Geometry check sheet. Reference: the model listing, model coordinates, mm. A direction names the side the tool comes from. Round coordinates to 2 decimals unless told otherwise and drop trailing zeros. Order: outer loops, then holes, each group sorted by start corner. A loop starts at its lowest first (then second) coordinate and runs counter-clockwise, first axis right, second up. Notation, with made-up numbers: (23, -33.75) - (30, -33.75) arc R22 ccw to (30, 3.25) - close; hole circle Ø10 at (83, 11). An arc over 180 degrees is marked (long way). Return JSON: item names as keys, results as strings. Group by question number.
Q1. Sectioned sample at B-B, the plane y = 1. Record the cut outline in (x, z).
Q2. Sectioned sample at A-A, the plane x = 0. Record the cut outline in (y, z) (3 decimals).
Q3. Tool access check on faces 1 (the flat face through (48.26, 0, 3)), 2 (the flat face through (1, -54.483, 3)), 3 (the flat face through (-61, 3.175, 3)). Record the directions out of +Z, -Z, +X, -X, +Y, -Y that give a thin tool (end or side, any length) a straight path to the whole face; none if there is none.
Q4. Draft check along Y on faces 4 (the cylindrical face through (0.62, -54.65, 3.13)), 5 (the flat face through (-39, 6, 6.35)), 6 (the cylindrical face through (-1.575, -73.643, 3.131)), 7 (the cylindrical face through (1.575, 73.643, 3.131)). Enter one of: pulls with the +Y half, pulls with the -Y half, needs draft (parallel to the pull), parting line crosses it, or undercut.
Q5. Sectioned sample at C-C, the plane x = -55.5. Record the cut outline in (y, z) (3 decimals).
Q6. Gauge pin test, flat ends, axial feed: pin 1 Ø5.5 at (x, y) = (0, -59.37) entering from -Z; pin 2 Ø1.9 at (x, z) = (16, 1.5) entering from +Y; pin 3 Ø1.9 at (x, z) = (-6.5, 3) entering from -Y; pin 4 Ø1.9 at (x, z) = (-55, 2) entering from -Y. Record the tip position at first contact, or that the pin passes through.
Q7. Material ranges on line 1 along X through (y, z) = (-1, 1.25); line 2 along X through (y, z) = (57, 2); line 3 along Y through (x, z) = (65, 1.75) (1 decimal), recorded low to high.
```python
from build123d import *

# Parameters (mm, degrees)
SKETCH1_R           = 73.66
BOSS_EXTRUDE1_DEPTH = 6.35
CUT_EXTRUDE1_DEPTH  = 7.35
SKETCH4_R           = 4.7625
CUT_EXTRUDE2_DEPTH  = 7.35
SKETCH5_W           = 76.2
SKETCH5_H           = 108.966
CUT_EXTRUDE5_DEPTH  = 7.35


with BuildPart() as part:
    # Sketch1 → Boss-Extrude1 (new body)
    with BuildSketch(Plane.XY):
        Circle(SKETCH1_R)
    extrude(amount=BOSS_EXTRUDE1_DEPTH)

    # Sketch2 → Cut-Extrude1 (cut, through all)
    with BuildSketch(Plane(origin=(0, 0, 0), x_dir=(-1, 0, 0), z_dir=(0, 0, -1))):
        Polygon((-48.26, 0), (-48.26, 3.175), (-76.2, 3.175), (-76.2, -3.175), (-48.26, -3.175), align=None)
        Polygon((48.26, -3.175), (48.26, 0), (48.26, 3.175), (76.2, 3.175), (76.2, -3.175), align=None)
    extrude(amount=-CUT_EXTRUDE1_DEPTH, mode=Mode.SUBTRACT)

    # Sketch4 → Cut-Extrude2 (cut, through all)
    with BuildSketch(Plane(origin=(0, 0, 0), x_dir=(-1, 0, 0), z_dir=(0, 0, -1))):
        with Locations((0, -59.3725)):
            Circle(SKETCH4_R)
        with Locations((0, 59.3725)):
            Circle(SKETCH4_R)
    extrude(amount=-CUT_EXTRUDE2_DEPTH, mode=Mode.SUBTRACT)

    # Sketch5 → Cut-Extrude5 (cut, through all)
    with BuildSketch(Plane(origin=(0, 0, 0), x_dir=(-1, 0, 0), z_dir=(0, 0, -1))):
        Rectangle(SKETCH5_W, SKETCH5_H)
    extrude(amount=-CUT_EXTRUDE5_DEPTH, mode=Mode.SUBTRACT)


solid = part.part
```
Reply:
{
 "1": {"outline": "(-48.26, 0) - (-38.1, 0) - (-38.1, 6.35) - (-48.26, 6.35) - close; (38.1, 0) - (48.26, 0) - (48.26, 6.35) - (38.1, 6.35) - close"},
 "2": {"outline": "(-73.66, 0) - (-64.135, 0) - (-64.135, 6.35) - (-73.66, 6.35) - close; (-54.61, 0) - (-54.483, 0) - (-54.483, 6.35) - (-54.61, 6.35) - close; (54.483, 0) - (54.61, 0) - (54.61, 6.35) - (54.483, 6.35) - close; (64.135, 0) - (73.66, 0) - (73.66, 6.35) - (64.135, 6.35) - close"},
 "3": {"face 1": "+Z, -Z, +X", "face 2": "+Z, -Z", "face 3": "+Z, -Z, -X"},
 "4": {"face 4": "undercut", "face 5": "needs draft", "face 6": "pulls with the -Y half", "face 7": "pulls with the +Y half"},
 "5": {"outline": "(-48.431, 0) - (-3.175, 0) - (-3.175, 6.35) - (-48.431, 6.35) - close; (3.175, 0) - (48.431, 0) - (48.431, 6.35) - (3.175, 6.35) - close"},
 "6": {"pin 1": "through", "pin 2": "y = 72.11", "pin 3": "y = -73.45", "pin 4": "y = -50.04"},
 "7": {"line 1": "-48.26 to -38.1, 38.1 to 48.26", "line 2": "-46.66 to -4.13, 4.13 to 46.66", "line 3": "-34.7 to -3.2, 3.2 to 34.7"}
}
